Read the model definition and answer for the solid it produces. Units are mm, in the model's axes. Coordinates: 2 decimals unless noted, no trailing zeros. Loops run counter-clockwise (first coordinate to the right, second up) from the corner with the lowest first, then second, coordinate; pieces in that order, holes last. Notation, with made-up numbers: (15.25, 57) -> (44.25, 57) arc R29 cw to (44.25, 91) -> close; hole circle Ø10 at (89, 77.5). An arc over 180 degrees is marked (long way). One line per question, with ' | ' between items. Start each with the question number.
```python
from build123d import *

# Parameters (mm, degrees)
SKETCH_1_W          = 6
SKETCH_1_H          = 41
EXTRUDE_1_DEPTH     = 16
SKETCH_2_R          = 1.75
CUT_EXTRUDE_1_DEPTH = 27.177280225
SKETCH_3_R          = 1.75
CUT_EXTRUDE_2_DEPTH = 27.68801229


with BuildPart() as part:
    # 草图1 → 凸台-拉伸1 (new body)
    with BuildSketch(Plane(origin=(0, 0, 0), x_dir=(1, 0, 0), z_dir=(0, 1, 0))):
        Rectangle(SKETCH_1_W, SKETCH_1_H)
    extrude(amount=EXTRUDE_1_DEPTH)

    # 草图2 → 切除-拉伸1 (cut, through all)
    with BuildSketch(Plane(origin=(0, 16, 0), x_dir=(1, 0, 0), z_dir=(0, 1, 0))):
        with Locations(Location((0, 13, 0), (0, 0, 270))):
            Circle(SKETCH_2_R)
        with Locations(Location((0, -13, 0), (0, 0, 270))):
            Circle(SKETCH_2_R)
    extrude(amount=-CUT_EXTRUDE_1_DEPTH, mode=Mode.SUBTRACT)

    # 草图3 → 切除-拉伸2 (cut, through all)
    with BuildSketch(Plane.ZY.offset(3)):
        with Locations((-17, 8)):
            Circle(SKETCH_3_R)
        with Locations((17, 8)):
            Circle(SKETCH_3_R)
    extrude(amount=-CUT_EXTRUDE_2_DEPTH, mode=Mode.SUBTRACT)


solid = part.part
```
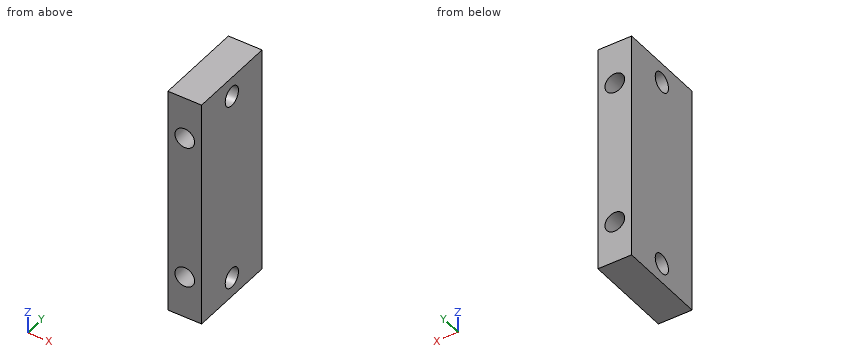
(1) Find the intervals of material crossed by probe 1 along Z at (x, y) = (2.2, 7.75); probe 2 along Y at (x, z) = (0.6, 17); probe 3 along Z at (x, y) = (-1.35, 1), in increasing order. Write a range as from..to.
(2) Section D-D on y = 1 is taken. Write down the section's boundary in (x, z), plus the area to 3 significant figures.
(3) Section C-C on z = -17 is taken. Write down the section's boundary in (x, y).
(4) Section A-A on y = 8 is taken. Write down the section's boundary in (x, z).
(5) This flat-tipped pin is pushed along its axis until it touches: pin 1 Ø1.5 at (x, z) = (0.5, -13.5) entering from +Y. Where does it stop, or does it pass through?
(6) Section B-B on x = -0.8 is taken. Write down the section's boundary in (y, z).
Working result:
1) probe 1: z = -20.5..-18.73, -15.27..15.27, 18.73..20.5 | probe 2: y = 0..6.25, 9.75..16 | probe 3: z = -20.5..-14.11, -11.89..11.89, 14.11..20.5
2) outline: (-3, -20.5) -> (3, -20.5) -> (3, 20.5) -> (-3, 20.5) -> close; hole circle Ø3.5 at (0, -13); hole circle Ø3.5 at (0, 13) | area: 227 mm2
3) outline: (-3, 0) -> (3, 0) -> (3, 6.25) -> (-3, 6.25) -> close; (-3, 9.75) -> (3, 9.75) -> (3, 16) -> (-3, 16) -> close
4) outline: (-3, -20.5) -> (3, -20.5) -> (3, -18.75) -> (-3, -18.75) -> close; (-3, -15.25) -> (3, -15.25) -> (3, 15.25) -> (-3, 15.25) -> close; (-3, 18.75) -> (3, 18.75) -> (3, 20.5) -> (-3, 20.5) -> close; hole circle Ø3.5 at (0, -13); hole circle Ø3.5 at (0, 13)
5) pin 1: passes through
6) outline: (0, -20.5) -> (16, -20.5) -> (16, -14.56) -> (0, -14.56) -> close; (0, -11.44) -> (16, -11.44) -> (16, 11.44) -> (0, 11.44) -> close; (0, 14.56) -> (16, 14.56) -> (16, 20.5) -> (0, 20.5) -> close; hole circle Ø3.5 at (8, -17); hole circle Ø3.5 at (8, 17)
